The listing builds one solid part. Answer for the finished solid, in the listing's coordinates (mm). A direction names the side the tool comes from. Give positions to 0.01 mm unless a question says otherwise; leave off trailing zeros. Write each loop counter-clockwise with the first axis right and the second up, starting at its lowest first coordinate (ties: lowest second). Pieces come first, ordered by that corner, then holes. Notation, with made-up numbers: (65, 43) - (108, 43) arc R20 ccw to (108, 70) - close; hole circle Ø8 at (51, 13). An arc over 180 degrees is marked (long way). Answer as CSV lines item,"result". Start each with the question number.
(1) Straight lines are drawn through the part: probe 1 along Y at (x, z) = (0, 5.1); probe 2 along Z at (x, y) = (-1, -3.75); probe 3 along Z at (x, y) = (10, 1.5). For each, find the intervals that lie inside material, in ascending order.
(2) Find section B-B (z = 3.4). State how many separate pieces and enclosed holes the cut face has, then the cut area to 3 significant figures.
(3) Find section A-A (x = -9.75). Write down the section's boundary in (y, z).
(4) For faces 1 (the face through (-8.763, -3.149, 4.014)), 2 (the face through (-1.3, 1.3, 3)), 3 (the face through (-3.746, 0.165, 5.296)), determine the directions among +Z, -Z, +X, -X, +Y, -Y from which every point of the face is accessible in a straight line to the end or side of a thin tool.
(5) For a pull along Y with two mould halves and no side action, classify faces 4 (the face through (0, -3, 0)), 5 (the face through (6.123, 2.689, 4.014)), 6 (the face through (-11.99, 0.53, 3.99)) as pulls with the +Y half, pulls with the -Y half, needs draft (parallel to the pull), parting line crosses it, or undercut.
(6) Find section D-D (y = -6.5). Write down the section's boundary in (x, z), then the cut area to 3 significant figures.
(7) Find section C-C (x = -7). Write down the section's boundary in (y, z), then the cut area to 3 significant figures.
(8) Each of these flat-tipped pins is pushed along its axis until it touches: pin 1 Ø2 at (x, y) = (9.51, -3.09) entering from -Z; pin 2 Ø2 at (x, y) = (9.51, 3.09) entering from +Z; pin 3 Ø3 at (x, z) = (7, 4.5) entering from +Y. Where does it stop, or does it pass through?
from build123d import *

# Parameters (mm, degrees)
ESQUISSE1_R                  = 4.5
BOSS_EXTRU_1_DEPTH           = 3
ESQUISSE2_R                  = 12
ESQUISSE2_R_2                = 1.4
BOSS_EXTRU_2_DEPTH           = 2
ESQUISSE3_R                  = 3.75
ESQUISSE3_R_2                = 1.4
BOSS_EXTRU_3_DEPTH           = 0.6
ESQUISSE4_R                  = 3
ENL_V_MAT_EXTRU_1_DEPTH      = 1.3
ESQUISSE5_R                  = 0.75
ENL_V_MAT_EXTRU_2_DEPTH      = 6
R_P_TITION_CIRCULAIRE1_COUNT = 20
ESQUISSE6_R                  = 0.75
ENL_V_MAT_EXTRU_3_DEPTH      = 6
R_P_TITION_CIRCULAIRE2_COUNT = 20


with BuildPart() as part:
    # Esquisse1 → Boss.-Extru.1 (new body)
    with BuildSketch(Plane.XY):
        Circle(ESQUISSE1_R)
        Polygon((2.011577371, -1.550856692), (2.011577371, -2.011577371), (1.550856692, -2.011577371), (1.541643286, -2.018647066), (1.4224, -2.463669069), (0.977377998, -2.344425783), (0.966648759, -2.348869979), (0.73628842, -2.747865791), (0.337292608, -2.517505451), (0.325778716, -2.519021284), (0, -2.8448), (-0.325778716, -2.519021284), (-0.337292608, -2.517505451), (-0.73628842, -2.747865791), (-0.966648759, -2.348869979), (-0.977377998, -2.344425783), (-1.4224, -2.463669069), (-1.541643286, -2.018647066), (-1.550856692, -2.011577371), (-2.011577371, -2.011577371), (-2.011577371, -1.550856692), (-2.018647066, -1.541643286), (-2.463669069, -1.4224), (-2.344425783, -0.977377998), (-2.348869979, -0.966648759), (-2.747865791, -0.73628842), (-2.517505451, -0.337292608), (-2.519021284, -0.325778716), (-2.8448, 0), (-2.519021284, 0.325778716), (-2.517505451, 0.337292608), (-2.747865791, 0.73628842), (-2.348869979, 0.966648759), (-2.344425783, 0.977377998), (-2.463669069, 1.4224), (-2.018647066, 1.541643286), (-2.011577371, 1.550856692), (-2.011577371, 2.011577371), (-1.550856692, 2.011577371), (-1.541643286, 2.018647066), (-1.4224, 2.463669069), (-0.977377998, 2.344425783), (-0.966648759, 2.348869979), (-0.73628842, 2.747865791), (-0.337292608, 2.517505451), (-0.325778716, 2.519021284), (0, 2.8448), (0.325778716, 2.519021284), (0.337292608, 2.517505451), (0.73628842, 2.747865791), (0.966648759, 2.348869979), (0.977377998, 2.344425783), (1.4224, 2.463669069), (1.541643286, 2.018647066), (1.550856692, 2.011577371), (2.011577371, 2.011577371), (2.011577371, 1.550856692), (2.018647066, 1.541643286), (2.463669069, 1.4224), (2.344425783, 0.977377998), (2.348869979, 0.966648759), (2.747865791, 0.73628842), (2.517505451, 0.337292608), (2.519021284, 0.325778716), (2.8448, 0), (2.519021284, -0.325778716), (2.517505451, -0.337292608), (2.747865791, -0.73628842), (2.348869979, -0.966648759), (2.344425783, -0.977377998), (2.463669069, -1.4224), (2.018647066, -1.541643286), align=None, mode=Mode.SUBTRACT)
    extrude(amount=BOSS_EXTRU_1_DEPTH)

    # Esquisse2 → Boss.-Extru.2 (add)
    with BuildSketch(Plane.XY.offset(3)):
        Circle(ESQUISSE2_R)
        Circle(ESQUISSE2_R_2, mode=Mode.SUBTRACT)
    extrude(amount=BOSS_EXTRU_2_DEPTH)

    # Esquisse3 → Boss.-Extru.3 (add)
    with BuildSketch(Plane.XY.offset(5)):
        Circle(ESQUISSE3_R)
        Circle(ESQUISSE3_R_2, mode=Mode.SUBTRACT)
    extrude(amount=BOSS_EXTRU_3_DEPTH)

    # Esquisse4 → Enlèv. mat.-Extru.1 (cut)
    with BuildSketch(Plane.XY.offset(5.6)):
        Circle(ESQUISSE4_R)
    extrude(amount=-ENL_V_MAT_EXTRU_1_DEPTH, mode=Mode.SUBTRACT)

    # Esquisse5 → Enlèv. mat.-Extru.2 (cut, through all)
    with BuildSketch(Plane.XY.offset(5)):
        with Locations((-10, 0)):
            Circle(ESQUISSE5_R)
        with Locations((-7, 0)):
            Circle(ESQUISSE5_R)
    enl_v_mat_extru_2 = extrude(amount=-ENL_V_MAT_EXTRU_2_DEPTH, mode=Mode.SUBTRACT)

    # Répétition circulaire1: Enlèv. mat.-Extru.2 ×20 about axis, 14 skipped
    r_p_tition_circulaire1_axis = Axis((0, 0, 0), (0, 0, 1))
    add([enl_v_mat_extru_2.rotate(r_p_tition_circulaire1_axis, i * 360 / R_P_TITION_CIRCULAIRE1_COUNT) for i in range(1, R_P_TITION_CIRCULAIRE1_COUNT) if i not in (2, 3, 4, 5, 6, 7, 8, 12, 13, 14, 15, 16, 17, 18)], mode=Mode.SUBTRACT)

    # Esquisse6 → Enlèv. mat.-Extru.3 (cut, through all)
    with BuildSketch(Plane.XY.offset(5)):
        with Locations((0, 8.5)):
            Circle(ESQUISSE6_R)
    enl_v_mat_extru_3 = extrude(amount=-ENL_V_MAT_EXTRU_3_DEPTH, mode=Mode.SUBTRACT)

    # Répétition circulaire2: Enlèv. mat.-Extru.3 ×20 about axis, 14 skipped
    r_p_tition_circulaire2_axis = Axis((0, 0, 0), (0, 0, 1))
    add([enl_v_mat_extru_3.rotate(r_p_tition_circulaire2_axis, i * 360 / R_P_TITION_CIRCULAIRE2_COUNT) for i in range(1, R_P_TITION_CIRCULAIRE2_COUNT) if i not in (2, 3, 4, 5, 6, 7, 8, 12, 13, 14, 15, 16, 17, 18)], mode=Mode.SUBTRACT)


solid = part.part
Result set:
1,probe 1,"-3.75 to -3, 3 to 3.75"
1,probe 2,"0 to 5"
1,probe 3,"3 to 5"
2,separate pieces,"1"
2,enclosed holes,"19"
2,area,"414 mm^2"
3,outline,"(-7, 3) - (-3.8, 3) - (-3.8, 5) - (-7, 5) - close; (-2.38, 3) - (-0.71, 3) - (-0.71, 5) - (-2.38, 5) - close; (0.71, 3) - (2.38, 3) - (2.38, 5) - (0.71, 5) - close; (3.8, 3) - (7, 3) - (7, 5) - (3.8, 5) - close"
4,face 1,"+Z, -Z"
4,face 2,"-Z"
4,face 3,"+Z"
5,face 4,"needs draft"
5,face 5,"undercut"
5,face 6,"parting line crosses it"
6,outline,"(-10.09, 3) - (10.09, 3) - (10.09, 5) - (-10.09, 5) - close"
6,area,"40.3 mm^2"
7,outline,"(-9.75, 3) - (-2.83, 3) - (-2.83, 5) - (-9.75, 5) - close; (-1.5, 3) - (-0.75, 3) - (-0.75, 5) - (-1.5, 5) - close; (0.75, 3) - (1.5, 3) - (1.5, 5) - (0.75, 5) - close; (2.83, 3) - (9.75, 3) - (9.75, 5) - (2.83, 5) - close"
7,area,"30.6 mm^2"
8,pin 1,"z = 3"
8,pin 2,"z = 5"
8,pin 3,"y = 10.67"
